Source: CAD feature listing. Evaluate the final solid. Frame: model axes, mm. Face numbers are marked on the shaded views. A direction names the side the tool comes from. Coordinates: 2 decimals unless noted, no trailing zeros. Write each loop counter-clockwise with the first axis right and the second up, starting at its lowest first coordinate (ties: lowest second). Pieces come first, ordered by that corner, then holes. Notation, with made-up numbers: (36, 19) - (72, 19) arc R16 ccw to (72, 50) - close; hole circle Ø10 at (23, 60). An arc over 180 degrees is marked (long way). One line per question, with ' | ' between items.
from build123d import *

# Parameters (mm, degrees)
SKETCH1_R           = 17.9
BOSS_EXTRUDE1_DEPTH = 50
SKETCH2_R           = 6.5
BOSS_EXTRUDE2_DEPTH = 4.5
SKETCH3_R           = 1.585
BOSS_EXTRUDE3_DEPTH = 12.5
SKETCH4_R           = 5.1
BOSS_EXTRUDE4_DEPTH = 3
BOSS_EXTRUDE5_START = 12.5
SKETCH5_R           = 1.585
BOSS_EXTRUDE5_DEPTH = 12.5
BOSS_EXTRUDE6_DEPTH = 8
SKETCH7_R           = 1.5
CUT_EXTRUDE1_DEPTH  = 8
CUT_EXTRUDE2_START  = -4.5
SKETCH8_R           = 1.585
CUT_EXTRUDE2_DEPTH  = 4.5
SKETCH9_R           = 1.585
CUT_EXTRUDE3_DEPTH  = 3.5


with BuildPart() as part:
    # Sketch1 → Boss-Extrude1 (new body)
    with BuildSketch(Plane(origin=(0, 0, 0), x_dir=(1, 0, 0), z_dir=(0, 1, 0))):
        with Locations(Location((0, 0, 0), (0, 0, 270))):
            Circle(SKETCH1_R)
    extrude(amount=BOSS_EXTRUDE1_DEPTH)

    # Sketch2 → Boss-Extrude2 (add)
    with BuildSketch(Plane(origin=(0, 50, 0), x_dir=(1, 0, 0), z_dir=(0, 1, 0))):
        with Locations(Location((0, 0, 0), (0, 0, 270))):
            Circle(SKETCH2_R)
    extrude(amount=BOSS_EXTRUDE2_DEPTH)

    # Sketch3 → Boss-Extrude3 (add)
    with BuildSketch(Plane(origin=(0, 54.5, 0), x_dir=(1, 0, 0), z_dir=(0, 1, 0))):
        with Locations(Location((0, 0, 0), (0, 0, 270))):
            Circle(SKETCH3_R)
    extrude(amount=BOSS_EXTRUDE3_DEPTH)

    # Sketch4 → Boss-Extrude4 (add)
    with BuildSketch(Plane.XZ):
        with Locations(Location((0, 0, 0), (0, 0, 90))):
            Circle(SKETCH4_R)
    extrude(amount=BOSS_EXTRUDE4_DEPTH)

    # Sketch5 → Boss-Extrude5 (add)
    with BuildSketch(Plane(origin=(0, -3, 0), x_dir=(-1, 0, 0), z_dir=(0, -1, 0)).offset(BOSS_EXTRUDE5_START)):
        with Locations(Location((0, 0, 0), (0, 0, 270))):
            Circle(SKETCH5_R)
    extrude(amount=-BOSS_EXTRUDE5_DEPTH)

    # Sketch6 → Boss-Extrude6 (add)
    with BuildSketch(Plane.XZ):
        Polygon((0, -13.95), (0, -13.7), (0, -13.45), (-0.5, -13.45), (-0.5, -13.95), align=None)
        Polygon((0, -13.45), (0, -13.7), (0, -13.95), (0.5, -13.95), (0.5, -13.45), align=None)
        Polygon((0, 13.45), (0, 13.7), (0, 13.95), (-0.5, 13.95), (-0.5, 13.45), align=None)
        Polygon((0, 13.95), (0, 13.7), (0, 13.45), (0.5, 13.45), (0.5, 13.95), align=None)
    extrude(amount=BOSS_EXTRUDE6_DEPTH)

    # Sketch7 → Cut-Extrude1 (cut)
    with BuildSketch(Plane(origin=(0, 50, 0), x_dir=(1, 0, 0), z_dir=(0, 1, 0))):
        with Locations(Location((12.5, 0, 0), (0, 0, 270))):
            Circle(SKETCH7_R)
        with Locations(Location((-12.5, 0, 0), (0, 0, 270))):
            Circle(SKETCH7_R)
    extrude(amount=-CUT_EXTRUDE1_DEPTH, mode=Mode.SUBTRACT)

    # Sketch8 → Cut-Extrude2 (cut)
    with BuildSketch(Plane(origin=(0, 67, 0), x_dir=(1, 0, 0), z_dir=(0, 1, 0)).offset(CUT_EXTRUDE2_START)):
        with Locations(Location((0, 0, 0), (0, 0, 270))):
            Circle(SKETCH8_R)
    extrude(amount=CUT_EXTRUDE2_DEPTH, mode=Mode.SUBTRACT)

    # Sketch9 → Cut-Extrude3 (cut)
    with BuildSketch(Plane.XZ.offset(15.5)):
        with Locations(Location((0, 0, 0), (0, 0, 270))):
            Circle(SKETCH9_R)
    extrude(amount=-CUT_EXTRUDE3_DEPTH, mode=Mode.SUBTRACT)


solid = part.part
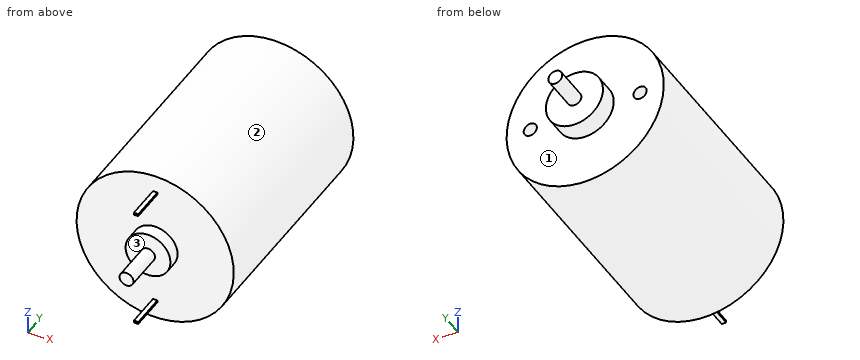
Item 1: Access query for the marked faces 1, 2 and 3. Directions: +Z, -Z, +X, -X, +Y, -Y. A direction counts if a zero-diameter tool reaches every point of the face in a straight line with its end or side. Return the directions, or none.
Check sheet entries:
face 1: +Y | face 2: +Y, -Y | face 3: -Y
Item 2: Cut plane D-D on x = 12.5. Return loops of the section in (y, z).
Check sheet entries:
outline: (0, -12.81) - (50, -12.81) - (50, -1.5) - (42, -1.5) - (42, 1.5) - (50, 1.5) - (50, 12.81) - (0, 12.81) - close
Item 3: Cut plane A-A on z = 0. Return loops of the section in (x, y) (3 decimals).
Check sheet entries:
outline: (-17.9, 0) - (-5.1, 0) - (-5.1, -3) - (-1.585, -3) - (-1.585, -12) - (1.585, -12) - (1.585, -3) - (5.1, -3) - (5.1, 0) - (17.9, 0) - (17.9, 50) - (14, 50) - (14, 42) - (11, 42) - (11, 50) - (6.5, 50) - (6.5, 54.5) - (1.585, 54.5) - (1.585, 62.5) - (-1.585, 62.5) - (-1.585, 54.5) - (-6.5, 54.5) - (-6.5, 50) - (-11, 50) - (-11, 42) - (-14, 42) - (-14, 50) - (-17.9, 50) - close
Item 4: Pin query (flat end, axial travel): pin 1 Ø6 at (x, z) = (-7.5, 5.5) entering from -Y; pin 2 Ø1.5 at (x, z) = (-12.5, 0.5) entering from +Y; pin 3 Ø3.5 at (x, z) = (12, -0.5) entering from +Y. Return the tip coordinate at first contact, or that it passes through.
Check sheet entries:
pin 1: y = 0 | pin 2: y = 42 | pin 3: y = 50
Item 5: Cut plane B-B on x = -3. Return loops of the section in (y, z).
Check sheet entries:
outline: (-3, -4.12) - (0, -4.12) - (0, -17.65) - (50, -17.65) - (50, -5.77) - (54.5, -5.77) - (54.5, 5.77) - (50, 5.77) - (50, 17.65) - (0, 17.65) - (0, 4.12) - (-3, 4.12) - close
Item 6: Cut plane C-C on y = 22. Return loops of the section in (x, z).
Check sheet entries:
outline: circle Ø35.8 at (0, 0)
Item 7: Ray query, line 1 along X through (y, z) = (45, 0); line 2 along Y through (x, z) = (-3.5, 7.5); line 3 along X through (y, z) = (24, 0). Return the intervals inside material, ascending. Write a range as [from, to].
Check sheet entries:
line 1: [-17.9, -14], [-11, 11], [14, 17.9] | line 2: [0, 50] | line 3: [-17.9, 17.9]
